Geometry check sheet. Reference: the model listing, model coordinates, mm. Coordinates: 2 decimals unless noted, no trailing zeros. Order: outer loops, then holes, each group sorted by start corner. A loop starts at its lowest first (then second) coordinate and runs counter-clockwise, first axis right, second up. Notation, with made-up numbers: (52, 27) - (90, 27) arc R30 cw to (90, 49) - close; hole circle Ø6 at (89.25, -8). An arc over 180 degrees is marked (long way). Put each result on its own line as item: value.
from build123d import *
from OCP.BRepFilletAPI import BRepFilletAPI_MakeChamfer

# Parameters (mm, degrees)
SKETCH_1_W               = 150
SKETCH_1_H               = 150
EXTRUDE_1_DEPTH          = 20
SKETCH_2_W               = 200
SKETCH_2_H               = 170
EXTRUDE_2_DEPTH          = 20
SKETCH_3_W               = 200
SKETCH_3_H               = 22.5
EXTRUDE_3_DEPTH          = 20
SKETCH_4_W               = 200
SKETCH_4_H               = 101.536616744
SKETCH_4_R               = 12
EXTRUDE_4_DEPTH          = 10
SKETCH_5_W               = 200
SKETCH_5_H               = 170
EXTRUDE_5_DEPTH          = 10
SKETCH_6_W               = 12.361111111
SKETCH_6_H               = 120
EXTRUDE_6_DEPTH          = 60
CHAMFER_1_SIZE           = 10
CHAMFER_1_SIZE2          = 12.546778674
SKETCH_8_R               = 12.5
CUT_EXTRUDE_1_DEPTH      = 200
SKETCH_9_R               = 5.6
CUT_EXTRUDE_2_DEPTH      = 200
FILLET_1_R               = 10
SKETCH_10_R              = 40
SKETCH_10_R_2            = 8.532995409
EXTRUDE_7_DEPTH          = 5
SKETCH_11_R              = 12.5
CUT_EXTRUDE_3_DEPTH      = 200
SKETCH_12_W              = 50
SKETCH_12_H              = 12.140710291
EXTRUDE_8_DEPTH          = 120
EXTRUDE_9_DEPTH          = 120
SKETCH_14_R              = 5
SKETCH_14_R_2            = 5.6
CUT_EXTRUDE_4_DEPTH      = 200
CUT_EXTRUDE_5_DEPTH      = 428.663313117
CUT_EXTRUDE_5_DEPTH_BACK = 428.663313117
SKETCH_16_W              = 64.88929467
SKETCH_16_H              = 154.650571828
SKETCH_17_R              = 25
SKETCH_17_R_2            = 12.5
EXTRUDE_11_DEPTH         = 8
RIB_1_REACH              = 411.018
SKETCH_18_WALL_W         = 895.028437604
SKETCH_18_WALL_H         = 15
CUT_EXTRUDE_6_DEPTH      = 428.663313117
CUT_EXTRUDE_6_DEPTH_BACK = 428.663313117
CUT_EXTRUDE_7_DEPTH      = 390.123413038
CUT_EXTRUDE_7_DEPTH_BACK = 390.123413038
SKETCH_20_W              = 77.763891656
SKETCH_20_H              = 49.195078016
CUT_EXTRUDE_8_DEPTH      = 361.312364484
CUT_EXTRUDE_8_DEPTH_BACK = 361.312364484
SKETCH_21_OUTSIDE_W      = 157.88
SKETCH_21_OUTSIDE_H      = 170.021
SKETCH_21_OUTSIDE_W_2    = 120.000001731
SKETCH_21_OUTSIDE_H_2    = 128.334009182
CUT_EXTRUDE_9_DEPTH      = 361.312364484
CUT_EXTRUDE_9_DEPTH_BACK = 361.312364484
SKETCH_22_R              = 12.5


with BuildPart() as part:
    # 草图1 → 凸台-拉伸1 (new body)
    with BuildSketch(Plane(origin=(0, 0, 0), x_dir=(1, 0, 0), z_dir=(0, 1, 0))):
        Rectangle(SKETCH_1_W, SKETCH_1_H)
    extrude(amount=EXTRUDE_1_DEPTH)

    # 草图2 → 凸台-拉伸2 (add)
    with BuildSketch(Plane(origin=(0, 20, 0), x_dir=(1, 0, 0), z_dir=(0, 1, 0))):
        with Locations((-25, 0)):
            Rectangle(SKETCH_2_W, SKETCH_2_H)
    extrude(amount=-EXTRUDE_2_DEPTH)

    # 草图3 → 凸台-拉伸3 (add)
    with BuildSketch(Plane(origin=(0, 20, 0), x_dir=(1, 0, 0), z_dir=(0, 1, 0))):
        with Locations((-25, -96.25)):
            Rectangle(SKETCH_3_W, SKETCH_3_H)
    extrude(amount=-EXTRUDE_3_DEPTH)

    # 草图4 → 凸台-拉伸4 (add)
    with BuildSketch(Plane(origin=(0, 20, 0), x_dir=(1, 0, 0), z_dir=(0, 1, 0))):
        with Locations((-25, -135.768308372)):
            Rectangle(SKETCH_4_W, SKETCH_4_H)
        with Locations(Location((35, -147.018308372, 0), (0, 0, 270))):
            Circle(SKETCH_4_R, mode=Mode.SUBTRACT)
        with Locations(Location((-85, -147.018308372, 0), (0, 0, 270))):
            Circle(SKETCH_4_R, mode=Mode.SUBTRACT)
    extrude(amount=EXTRUDE_4_DEPTH)

    # 草图5 → 凸台-拉伸5 (add)
    with BuildSketch(Plane(origin=(0, 20, 0), x_dir=(1, 0, 0), z_dir=(0, 1, 0))):
        with Locations((-25, 0)):
            Rectangle(SKETCH_5_W, SKETCH_5_H)
    extrude(amount=EXTRUDE_5_DEPTH)

    # 草图6 → 凸台-拉伸6 (add, symmetric)
    with BuildSketch(Plane(origin=(-25, 0, 0), x_dir=(0, 0, -1), z_dir=(1, 0, 0))):
        Polygon((-67.5, 30), (-5, 30), (-42.777777778, 230), (-67.5, 230), align=None)
        with Locations((-61.319444445, 290)):
            Rectangle(SKETCH_6_W, SKETCH_6_H)
    extrude(amount=EXTRUDE_6_DEPTH, both=True)

    # 倒角1: one chamfer whose edges measure the first distance from different faces: ONE call of the kernel's chamfer builder (chamfer() names one face for all edges)
    chamfer_1_edges_1 = [part.edges().sort_by_distance(p)[0] for p in [
        (-85, 30, 36.25),
        (-25, 30, 67.5),
        (35, 30, 36.25),
    ]]
    chamfer_1_edges_2 = [part.edges().sort_by_distance(p)[0] for p in [
        (-25, 30, 5),
    ]]
    chamfer_1_side_2 = [part.faces().sort_by_distance(p)[0] for p in [
        (-121.627580479, 30, 50.768308372),
    ]]
    chamfer_1 = BRepFilletAPI_MakeChamfer(part.part.solid().wrapped)
    for e in chamfer_1_edges_1:
        chamfer_1.Add(CHAMFER_1_SIZE, e.wrapped)
    for e in chamfer_1_edges_2:
        chamfer_1.Add(CHAMFER_1_SIZE, CHAMFER_1_SIZE2, e.wrapped, chamfer_1_side_2[0].wrapped)  # the first distance lies on this face
    add(Compound.cast(chamfer_1.Shape()), mode=Mode.REPLACE)

    # 草图8 → 切除-拉伸1 (cut)
    with BuildSketch(Plane.XY.offset(67.5)):
        with Locations((-25, 285.8)):
            Circle(SKETCH_8_R)
    extrude(amount=-CUT_EXTRUDE_1_DEPTH, mode=Mode.SUBTRACT)

    # 草图9 → 切除-拉伸2 (cut)
    with BuildSketch(Plane.XY.offset(67.5)):
        with Locations((-72.14, 333.54)):
            Circle(SKETCH_9_R)
        with Locations((-72.14, 239.26)):
            Circle(SKETCH_9_R)
        with Locations((22.14, 239.26)):
            Circle(SKETCH_9_R)
        with Locations((22.14, 333.54)):
            Circle(SKETCH_9_R)
    extrude(amount=-CUT_EXTRUDE_2_DEPTH, mode=Mode.SUBTRACT)

    # 圆角1
    fillet_1_edges = [part.edges().sort_by_distance(p)[0] for p in [
        (35, 350, 61.319444444),
        (-85, 350, 61.319444444),
    ]]
    fillet(fillet_1_edges, radius=FILLET_1_R)

    # 草图10 → 凸台-拉伸7 (add)
    with BuildSketch(Plane.XY.offset(67.5)):
        with Locations((-25, 285.8)):
            Circle(SKETCH_10_R)
        with Locations((-25, 285.8)):
            Circle(SKETCH_10_R_2, mode=Mode.SUBTRACT)
    extrude(amount=EXTRUDE_7_DEPTH)

    # 草图11 → 切除-拉伸3 (cut)
    with BuildSketch(Plane.XY.offset(72.5)):
        with Locations((-25, 285.8)):
            Circle(SKETCH_11_R)
    extrude(amount=-CUT_EXTRUDE_3_DEPTH, mode=Mode.SUBTRACT)

    # 草图12 → 凸台-拉伸8 (add)
    with BuildSketch(Plane(origin=(35, 0, 0), x_dir=(0, 0, -1), z_dir=(1, 0, 0))):
        with Locations((-67.777777778, 223.929644855)):
            Rectangle(SKETCH_12_W, SKETCH_12_H)
    extrude(amount=-EXTRUDE_8_DEPTH)

    # 草图13 → 凸台-拉伸9 (add)
    with BuildSketch(Plane(origin=(35, 0, 0), x_dir=(0, 0, -1), z_dir=(1, 0, 0))):
        Polygon((-92.777777778, 230), (-102.486640647, 230), (-102.486640647, 350), (-112.486640647, 350), (-112.486640647, 230), (-112.486640647, 217.859289709), (-92.777777778, 217.859289709), align=None)
    extrude(amount=-EXTRUDE_9_DEPTH)

    # 草图14 → 切除-拉伸4 (cut)
    with BuildSketch(Plane.XY.offset(112.486640647)):
        with Locations((22.14, 332.94)):
            Circle(SKETCH_14_R)
        with Locations((22.14, 238.66)):
            Circle(SKETCH_14_R_2)
        with Locations((-72.14, 238.66)):
            Circle(SKETCH_14_R_2)
        with Locations((-72.14, 332.94)):
            Circle(SKETCH_14_R_2)
    extrude(amount=-CUT_EXTRUDE_4_DEPTH, mode=Mode.SUBTRACT)

    # 草图16 → 切除-拉伸5 (cut, two sides: drawn at the far end of the back side and taken through both)
    with BuildSketch(Plane.ZY.offset(85).offset(-CUT_EXTRUDE_5_DEPTH_BACK)):
        with Locations((49.451016332, 307.325285914)):
            Rectangle(SKETCH_16_W, SKETCH_16_H)
    extrude(amount=CUT_EXTRUDE_5_DEPTH + CUT_EXTRUDE_5_DEPTH_BACK, mode=Mode.SUBTRACT)

    # 草图17 → 凸台-拉伸11 (add)
    with BuildSketch(Plane.XY.offset(112.486640647)):
        with Locations((-24.999999135, 285.832995409)):
            Circle(SKETCH_17_R)
        with Locations((-24.999999135, 285.832995409)):
            Circle(SKETCH_17_R_2, mode=Mode.SUBTRACT)
    extrude(amount=EXTRUDE_11_DEPTH)

    # 草图18 wall → 筋1 (add, up to next)
    with BuildSketch(Plane(origin=(-25, 187.859289709, 89.993320324), x_dir=(0, -0.800085500873, -0.599885981911), z_dir=(0, 0.599885981911, -0.800085500873)), mode=Mode.PRIVATE) as rib_1_sk1:
        Rectangle(SKETCH_18_WALL_W, SKETCH_18_WALL_H)
    rib_1_tool1 = extrude(rib_1_sk1.sketch, amount=RIB_1_REACH, mode=Mode.PRIVATE) - part.part
    add(rib_1_tool1.solids().sort_by_distance((-25, 187.859289709, 89.993320324))[0])

    # 草图19 → 切除-拉伸6 (cut, two sides: drawn at the far end of the back side and taken through both)
    with BuildSketch(Plane(origin=(35, 0, 0), x_dir=(0, 0, -1), z_dir=(1, 0, 0)).offset(-CUT_EXTRUDE_6_DEPTH_BACK)):
        Polygon((-112.486640647, 217.859289709), (203.167671069, 217.859289709), (203.167671069, -23.133322037), (-112.486640647, -23.133322037), (-240.759412705, -23.133322037), (-240.759412705, 217.859289709), align=None)
    extrude(amount=CUT_EXTRUDE_6_DEPTH + CUT_EXTRUDE_6_DEPTH_BACK, mode=Mode.SUBTRACT)

    # 草图20 → 切除-拉伸7 (cut, two sides: drawn at the far end of the back side and taken through both)
    with BuildSketch(Plane(origin=(35, 0, 0), x_dir=(0, 0, -1), z_dir=(1, 0, 0)).offset(-CUT_EXTRUDE_7_DEPTH_BACK)):
        with Locations((-63.604694819, 225.128578756)):
            Rectangle(SKETCH_20_W, SKETCH_20_H)
    extrude(amount=CUT_EXTRUDE_7_DEPTH + CUT_EXTRUDE_7_DEPTH_BACK, mode=Mode.SUBTRACT)

    # 草图21 outside → 切除-拉伸8 (cut, two sides: drawn at the far end of the back side and taken through both)
    with BuildSketch(Plane.XY.offset(112.486640647).offset(-CUT_EXTRUDE_8_DEPTH_BACK)):
        with Locations((-25, 283.9295)):
            Rectangle(SKETCH_21_OUTSIDE_W, SKETCH_21_OUTSIDE_H)
        with Locations((-24.999999134, 285.832995409)):
            Rectangle(SKETCH_21_OUTSIDE_W_2, SKETCH_21_OUTSIDE_H_2, mode=Mode.SUBTRACT)
    extrude(amount=CUT_EXTRUDE_8_DEPTH + CUT_EXTRUDE_8_DEPTH_BACK, mode=Mode.SUBTRACT)

    # 草图22 → 切除-拉伸9 (cut, two sides: drawn at the far end of the back side and taken through both)
    with BuildSketch(Plane.XY.offset(112.486640647).offset(-CUT_EXTRUDE_9_DEPTH_BACK)):
        with Locations((-24.999999135, 285.832995409)):
            Circle(SKETCH_22_R)
    extrude(amount=CUT_EXTRUDE_9_DEPTH + CUT_EXTRUDE_9_DEPTH_BACK, mode=Mode.SUBTRACT)


solid = part.part
Q1. Section check A-A on x = -72.14. Record the boundary of the cut face in (y, z).
Answer block:
outline: (221.67, 102.49) - (233.06, 102.49) - (233.06, 112.49) - (221.67, 112.49) - close; (244.26, 102.49) - (327.34, 102.49) - (327.34, 112.49) - (244.26, 112.49) - close; (338.54, 102.49) - (350, 102.49) - (350, 112.49) - (338.54, 112.49) - close
Q2. Section check B-B on y = 238.66. Record the boundary of the cut face in (x, z), then the cut area to 3 significant figures.
Answer block:
outline: (-85, 102.49) - (-77.74, 102.49) - (-77.74, 112.49) - (-85, 112.49) - close; (-66.54, 102.49) - (16.54, 102.49) - (16.54, 112.49) - (-66.54, 112.49) - close; (27.74, 102.49) - (35, 102.49) - (35, 112.49) - (27.74, 112.49) - close
area: 976 mm^2
Q3. Section check D-D on y = 276. Record the boundary of the cut face in (x, z), then the cut area to 3 significant figures.
Answer block:
outline: (-85, 102.49) - (-32.72, 102.49) - (-32.72, 120.49) - (-47.99, 120.49) - (-47.99, 112.49) - (-85, 112.49) - close; (-17.28, 102.49) - (35, 102.49) - (35, 112.49) - (-2.01, 112.49) - (-2.01, 120.49) - (-17.28, 120.49) - close
area: 1,290 mm^2
Q4. Thickness scan on L1, parallel to Y at x = -72.14, z = 107.75; L2, parallel to Y at x = -25, z = 108.5; L3, parallel to Z at x = 1.5, y = 299. Record the ranges inside material, lowest first. Write a range as [from, to].
Answer block:
L1: y = [221.67, 233.06], [244.26, 327.34], [338.54, 350]
L2: y = [221.67, 273.33], [298.33, 350]
L3: z = [102.49, 112.49]
Q5. Section check C-C on x = -25. Record the boundary of the cut face in (y, z), then the cut area to 3 significant figures.
Answer block:
outline: (221.67, 102.49) - (273.33, 102.49) - (273.33, 120.49) - (260.83, 120.49) - (260.83, 112.49) - (221.67, 112.49) - close; (298.33, 102.49) - (350, 102.49) - (350, 112.49) - (310.83, 112.49) - (310.83, 120.49) - (298.33, 120.49) - close
area: 1,230 mm^2
Q6. Draft check along X on faces 1 (the flat face through (35, 287, 108)), 2 (the cylindrical face through (24.828, 337.156, 107.557)), 3 (the flat face through (-51, 287, 112.487)), 4 (the cylindrical face through (-28.25, 310.62, 116.43)). Enter one of: pulls with the +X half, pulls with the -X half, needs draft (parallel to the pull), parting line crosses it, or undercut.
Answer block:
face 1: pulls with the +X half
face 2: undercut
face 3: needs draft
face 4: parting line crosses it
Q7. Depth check by flat-ended pin: pin 1 Ø9 at (x, y) = (22.14, 238.66) entering from -Z; pin 2 Ø13 at (x, y) = (22.14, 332.94) entering from -Z; pin 3 Ø6 at (x, y) = (16.5, 283.5) entering from +Z. Enter the tip coordinate at first touch or a pass-through.
Answer block:
pin 1: passes through
pin 2: stops at z = 102.49
pin 3: stops at z = 112.49
